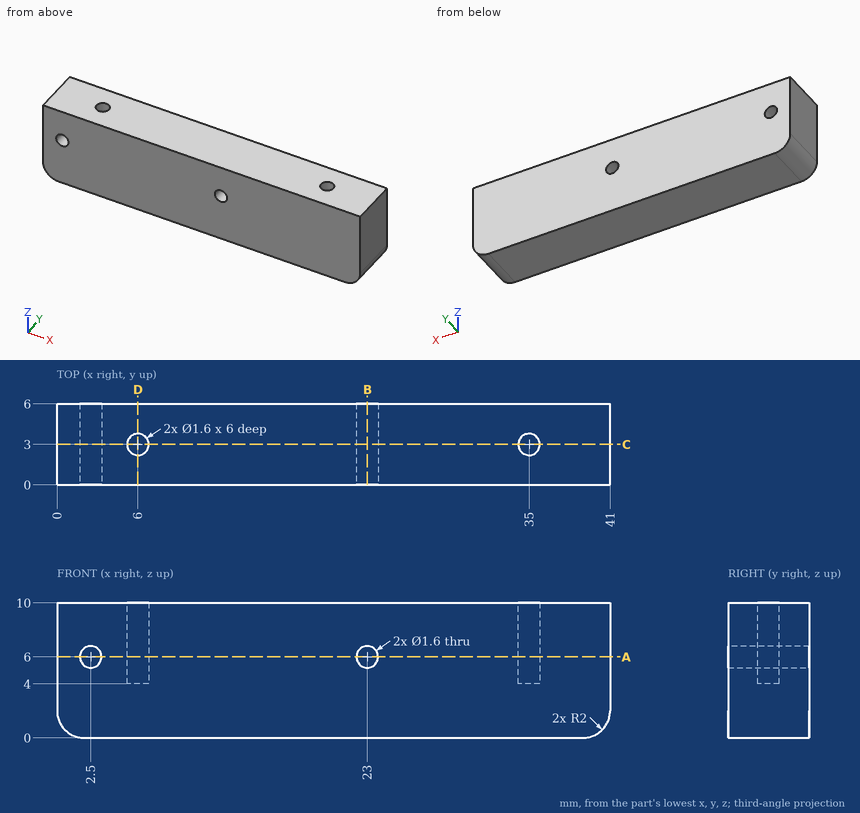
Geometry check sheet. Reference: drawing and pictorial views, mm from the part's lowest x, y, z. Give positions to 0.01 mm unless a question says otherwise; leave off trailing zeros. Write each loop counter-clockwise with the first axis right and the second up, starting at its lowest first coordinate (ties: lowest second). Pieces come first, ordered by that corner, then holes. Notation, with made-up numbers: (71.25, -39) -> (87.25, -39) arc R27 cw to (87.25, -20) -> close; hole circle Ø3 at (8, 50). An arc over 180 degrees is marked (long way). One line per item, written item: value. Start each with the question number.
Item 1: Section check D-D on x = 6. Record the cut outline in (y, z), then the cut area to 3 significant figures.
Item 2: Section check C-C on y = 3. Record the cut outline in (x, z), then the cut area to 3 significant figures.
Item 3: Section check B-B on x = 23. Record the cut outline in (y, z), then the cut area to 3 significant figures.
Item 4: Section check A-A on z = 6. Record the cut outline in (x, y).
Item 5: Material ranges on probe 1 along Z at (x, y) = (23, 1.45); probe 2 along Y at (x, z) = (6, 8); probe 3 along X at (y, z) = (3.65, 6), recorded low to high. Write a range as from..to.
Item 6: Gauge pin test, flat ends, axial feed: pin 1 (1.3 mm diameter, centred on x = 35, y = 3, fed in from +Z); pin 2 (1.4 mm diameter, centred on x = 2.5, z = 6, fed in from +Y). Record the tip position at first contact, or that the pin passes through.
Results list:
1. outline: (0, 0) -> (6, 0) -> (6, 10) -> (3.8, 10) -> (3.8, 4) -> (2.2, 4) -> (2.2, 10) -> (0, 10) -> close
1. area: 50.4 mm²
2. outline: (0, 2) arc R2 ccw to (2, 0) -> (39, 0) arc R2 ccw to (41, 2) -> (41, 10) -> (35.8, 10) -> (35.8, 4) -> (34.2, 4) -> (34.2, 10) -> (6.8, 10) -> (6.8, 4) -> (5.2, 4) -> (5.2, 10) -> (0, 10) -> close; hole circle Ø1.6 at (2.5, 6); hole circle Ø1.6 at (23, 6)
2. area: 385 mm²
3. outline: (0, 0) -> (6, 0) -> (6, 5.2) -> (0, 5.2) -> close; (0, 6.8) -> (6, 6.8) -> (6, 10) -> (0, 10) -> close
3. area: 50.4 mm²
4. outline: (0, 0) -> (1.7, 0) -> (1.7, 6) -> (0, 6) -> close; (3.3, 0) -> (22.2, 0) -> (22.2, 6) -> (3.3, 6) -> close; (23.8, 0) -> (41, 0) -> (41, 6) -> (23.8, 6) -> close; hole circle Ø1.6 at (6, 3); hole circle Ø1.6 at (35, 3)
5. probe 1: 0..5.2, 6.8..10
5. probe 2: 0..2.2, 3.8..6
5. probe 3: 0..1.7, 3.3..5.53, 6.47..22.2, 23.8..34.53, 35.47..41
6. pin 1: z = 4
6. pin 2: through
